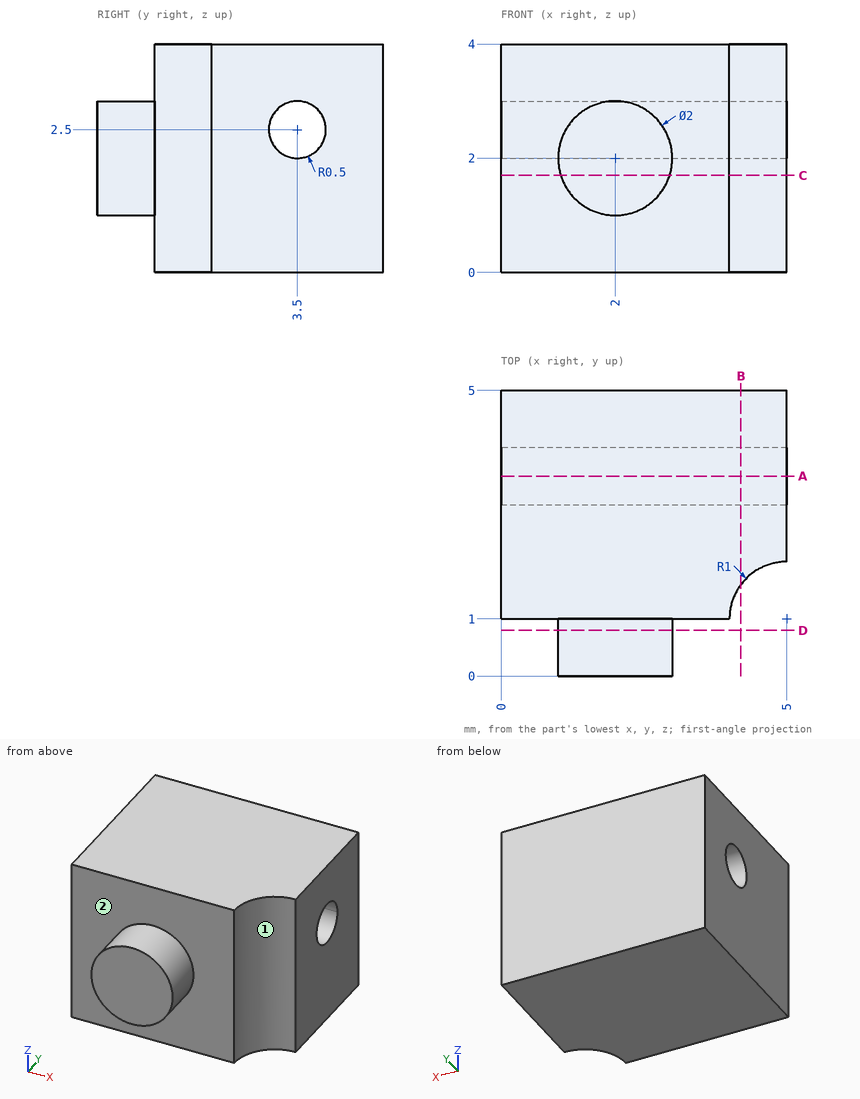
Design review of the part shown in the three views and the two pictorial views. Dimensions are in mm from the part's minimum x, y and z. A direction names the side the tool comes from. Coordinates: 2 decimals unless noted, no trailing zeros. Loops run counter-clockwise (first coordinate to the right, second up) from the corner with the lowest first, then second, coordinate; pieces in that order, holes last.
(1) Consider section A-A, the plane y = 3.5. Give the boundary of the cut face in (x, z).
Determined:
outline: (0, 0) - (5, 0) - (5, 2) - (0, 2) - close; (0, 3) - (5, 3) - (5, 4) - (0, 4) - close
(2) Tool access review of the marked faces 1 and 2: name each direction out of +Z, -Z, +X, -X, +Y, -Y from which nothing blocks a thin tool from reaching the whole face with its end or side.
Determined:
face 1: +Z, -Z, +X, -Y
face 2: -Y
(3) Wall thickness on L1, parallel to Y at x = 2.9, z = 0.6; L2, parallel to Y at x = 2.7, z = 2.85; L3, parallel to Y at x = 2.6, z = 2.3: over which ranges is each line inside the solid? List them lowest first.
Determined:
L1: y = 1 to 5
L2: y = 1 to 3.14, 3.86 to 5
L3: y = 0 to 3.04, 3.96 to 5
(4) Consider section D-D, the plane y = 0.8. Give the boundary of the cut face in (x, z), plus the area to 3 significant figures.
Determined:
outline: circle Ø2 at (2, 2)
area: 3.14 mm2
(5) Consider section B-B, the plane x = 4.2. Give the boundary of the cut face in (y, z).
Determined:
outline: (1.6, 0) - (5, 0) - (5, 4) - (1.6, 4) - close; hole (3.85, 2.85) arc R0.5 ccw (long way) to (4, 2.5) arc R0.5 ccw to start
(6) Consider section C-C, the plane z = 1.7. Give the boundary of the cut face in (x, y), plus the area to 3 significant figures.
Determined:
outline: (0, 1) - (1.05, 1) - (1.05, 0) - (2.95, 0) - (2.95, 1) - (4, 1) arc R1 cw to (5, 2) - (5, 5) - (0, 5) - close
area: 21.1 mm2
